```python
from build123d import *

# Parameters (mm, degrees)
F0_W     = 50
F0_H     = 50
F0_W_2   = 40
F0_H_2   = 40
F1_DEPTH = 140
F2_SIZE  = 3


with BuildPart() as f1:
    # F0 (on Top) → F1 (new body)
    with BuildSketch(Plane.XY):
        Rectangle(F0_W, F0_H)
        Rectangle(F0_W_2, F0_H_2, mode=Mode.SUBTRACT)
    extrude(amount=F1_DEPTH)

    # F2
    f2_edges = [f1.edges().sort_by_distance(p)[0] for p in [
        (25, -25, 70),
        (-25, -25, 70),
        (25, 25, 70),
        (-25, 25, 70),
    ]]
    chamfer(f2_edges, length=F2_SIZE)


solid = f1.part
```
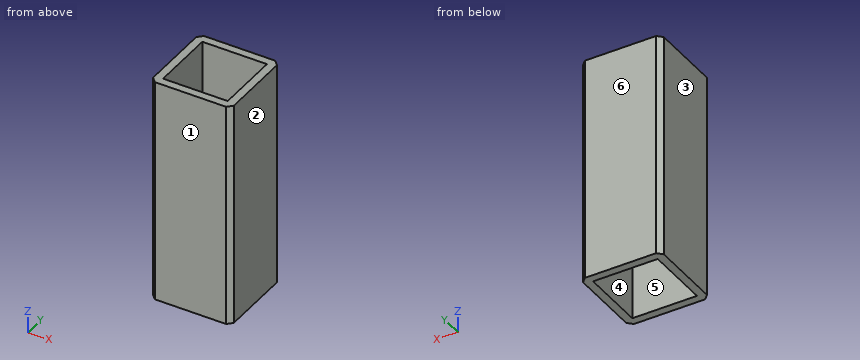
Verification items for the finished model (mm, model axes). Face numbers are marked on the shaded views. A direction names the side the tool comes from. Round coordinates to 2 decimals unless told otherwise and drop trailing zeros. Write each loop counter-clockwise with the first axis right and the second up, starting at its lowest first coordinate (ties: lowest second). Pieces come first, ordered by that corner, then holes.
1. Section check C-C on z = 127.5. Enter the section's corners in (x, y), plus the area to 3 significant figures.
2. Access from +Z, -Z, +X, -X, +Y, -Y to the whole of each face (thin tool, end or side, straight path). Record for the marked faces 5 and 6.
3. Draft check along X on the marked faces 1, 2, 3 and 4. Enter one of: +X half, -X half, draft (parallel to the pull), parting line (faces both ways), or undercut.
4. Section check A-A on y = -1. Enter the section's corners in (x, z).
5. Scan lines: L1, parallel to Y at x = -18.5, z = 111.5; L2, parallel to X at y = 22.5, z = 81. Record each from-to range of solid material in increasing order.
Answer:
1. outline: (-25, -22) - (-22, -25) - (22, -25) - (25, -22) - (25, 22) - (22, 25) - (-22, 25) - (-25, 22) - close; hole (-20, -20) - (20, -20) - (20, 20) - (-20, 20) - close
1. area: 882 mm2
2. face 5: +Z, -Z
2. face 6: +Z, -Z, +X, -X, +Y
3. face 1: draft
3. face 2: +X half
3. face 3: -X half
3. face 4: undercut
4. outline: (-25, 0) - (-20, 0) - (-20, 140) - (-25, 140) - close; (20, 0) - (25, 0) - (25, 140) - (20, 140) - close
5. L1: y = -25 to -20, 20 to 25
5. L2: x = -24.5 to 24.5
